from build123d import *

# Parameters (mm, degrees)
SKETCH1_W           = 50.8
SKETCH1_H           = 30.5
SKETCH1_W_2         = 48.4
SKETCH1_H_2         = 28.1
BOSS_EXTRUDE1_DEPTH = 462
SKETCH2_R           = 2
CUT_EXTRUDE1_DEPTH  = 464.701854644


with BuildPart() as part:
    # Sketch1 → Boss-Extrude1 (new body)
    with BuildSketch(Plane(origin=(0, 0, 0), x_dir=(1, 0, 0), z_dir=(0, 1, 0))):
        Rectangle(SKETCH1_W, SKETCH1_H)
        Rectangle(SKETCH1_W_2, SKETCH1_H_2, mode=Mode.SUBTRACT)
    extrude(amount=BOSS_EXTRUDE1_DEPTH)

    # Sketch2 → Cut-Extrude1 (cut, through all)
    with BuildSketch(Plane(origin=(0, 0, -15.25), x_dir=(-1, 0, 0), z_dir=(0, 0, -1))):
        with Locations((0, 231)):
            Circle(SKETCH2_R)
        with Locations((0, 381)):
            Circle(SKETCH2_R)
        with Locations((0, 81)):
            Circle(SKETCH2_R)
    extrude(amount=-CUT_EXTRUDE1_DEPTH, mode=Mode.SUBTRACT)


solid = part.part
Build history of the part. All positions in model axes, mm. A direction names the side the tool comes from. Coordinates: 2 decimals unless noted, no trailing zeros. Write each loop counter-clockwise with the first axis right and the second up, starting at its lowest first coordinate (ties: lowest second). Pieces come first, ordered by that corner, then holes.
(1) Mould opens along Z. For faces 1 (the flat face through (0, 228, 14.05)), 2 (the flat face through (-2, 0, 15)), 3 (the flat face through (0, 228, -14.05)), 4 (the flat face through (0, 228, -15.25)) say: pulls with the +Z half, pulls with the -Z half, needs draft (parallel to the pull), parting line crosses it, or undercut.
(2) Cut at A-A on x = -14.5. List the corners of the cut face in (y, z), and give its area (3 significant figures).
(3) Drill centre lines: line 1 (Z direction, x = 23, y = 308.5); line 2 (X direction, y = 381, z = 14.8); line 3 (X direction, y = 228.5, z = 13). Where is each one in solid material? Low to high.
(4) 3-axis set-ups, long thin cutter, end or side, ignore diameter. For faces 5 (the flat face through (24.2, 228, 0)), 6 (the flat face through (-2, 462, 15)): which of +Z, -Z, +X, -X, +Y, -Y reach the whole face in a straight line?
(5) Cut at B-B on y = 189.5. List the corners of the cut face in (x, z).
(6) Pin check, flat tip, straight feed: pin 1 Ø2.5 at (x, y) = (0, 381) entering from -Z. Stop position of the tip, or through.
(7) Cut at C-C on z = -0.5. List the corners of the cut face in (x, y), and give its area (3 significant figures).
Working result:
1. face 1: undercut
1. face 2: needs draft
1. face 3: undercut
1. face 4: pulls with the -Z half
2. outline: (0, -15.25) - (462, -15.25) - (462, -14.05) - (0, -14.05) - close; (0, 14.05) - (462, 14.05) - (462, 15.25) - (0, 15.25) - close
2. area: 1,110 mm2
3. line 1: z = -15.25 to -14.05, 14.05 to 15.25
3. line 2: x = -25.4 to -2, 2 to 25.4
3. line 3: x = -25.4 to -24.2, 24.2 to 25.4
4. face 5: +Y, -Y
4. face 6: +Z, -Z, +X, -X, +Y
5. outline: (-25.4, -15.25) - (25.4, -15.25) - (25.4, 15.25) - (-25.4, 15.25) - close; hole (-24.2, -14.05) - (24.2, -14.05) - (24.2, 14.05) - (-24.2, 14.05) - close
6. pin 1: passes through
7. outline: (-25.4, 0) - (-24.2, 0) - (-24.2, 462) - (-25.4, 462) - close; (24.2, 0) - (25.4, 0) - (25.4, 462) - (24.2, 462) - close
7. area: 1,110 mm2
